Autodesk Inventor part; units mm, degrees
ref_plane "YZ Plane" through (0, 0, 0) normal (1, 0, 0) x (0, 1, 0)
ref_plane "XZ Plane" through (0, 0, 0) normal (0, 1, 0) x (-1, 0, 0)
ref_plane "XY Plane" through (0, 0, 0) normal (0, 0, 1) x (1, 0, 0)
sketch "Sketch1" plane through (0, 0, 0) normal (1, 0, 0) x (0, 1, 0)
  line L0 (0, 20) -> (6, 20) construction
  arc A0 (7.7498, 0) -> (6, 20) centre (-30.6677, 6.7154) ccw construction
  line L1 (0, 16) -> (0, 0) construction
  line L2 (6, 20) -> (2.4961, 20) construction
  line L3 (7.7498, 0) -> (4.5, 0) construction
  line L4 (4.5, 10) -> (0, 10)
  line L5 (4.5, 10) -> (4.5, 0)
  line L6 (0, 16) -> (0, 10)
  line L7 (7.7498, 0) -> (6, 20) construction
  line L8 (4.5, 0) -> (7.7498, 0)
  line L9 (7.7498, 0) -> (6, 20)
  line L10 (0, 16) -> (0.8, 16)
  line L11 (0.8, 16) -> (0.8, 20)
  line L12 (0.8, 20) -> (6, 20)
  dimension "d0" = 6
  dimension "d5" = 4.5
  dimension "d11" = 10
  dimension "d12" = 20
  dimension "d13" = 95
  dimension "d21" = 4
  dimension "d22" = 0.8
revolve "Revolution1" add sketch "Sketch1" angle 360 about axis through (0, 0, 16) along (0, 0, -1)
properties part number "brush fitting parta v4"
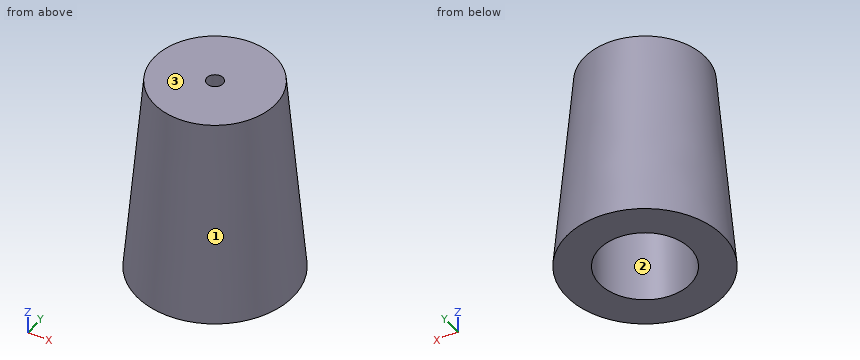
Design review of the part built by this model. Coordinates are the model's own, in mm. Face numbers are marked on the shaded views. Coordinates: 2 decimals unless noted, no trailing zeros. Order: outer loops, then holes, each group sorted by start corner. A loop starts at its lowest first (then second) coordinate and runs counter-clockwise, first axis right, second up.
1) Mouldability with a two-part tool opening along X and no side actions: class the marked faces 1, 2 and 3 as +X half, -X half, draft (parallel to the pull), parting line (faces both ways), or undercut.
2) Wall thickness on line 1 along Z through (x, y) = (1.5, 1.25); line 2 along X through (y, z) = (0, 18.6); line 3 along X through (y, z) = (0.5, 5.5): over which ranges is each line inside the solid? List them lowest first.
3) Take a section at A-A, the plane x = 0. Give the boundary of the cut face in (y, z), and give its area (3 significant figures).
4) Clearance check with flat-ended pins moving along their axes: pin 1 (1.5 mm diameter, centred on x = -6, z = 17, fed in from -Y); pin 2 (2 mm diameter, centred on x = -4.5, z = 6.5, fed in from +Y); pin 3 (2 mm diameter, centred on x = -3, z = 6.5, fed in from +Y). State where each tip first meets the part, or that it passes through.
5) Take a section at C-C, the plane z = 1.75. Give the boundary of the cut face in (x, y), and give its area (3 significant figures).
6) Take a section at D-D, the plane z = 18.5. Give the boundary of the cut face in (x, y), and give its area (3 significant figures).
Returned:
1. face 1: parting line
1. face 2: undercut
1. face 3: draft
2. line 1: z = 10 to 20
2. line 2: x = -6.12 to -0.8, 0.8 to 6.12
2. line 3: x = -7.25 to -4.47, 4.47 to 7.25
3. outline: (-7.75, 0) - (-4.5, 0) - (-4.5, 10) - (4.5, 10) - (4.5, 0) - (7.75, 0) - (6, 20) - (0.8, 20) - (0.8, 16) - (-0.8, 16) - (-0.8, 20) - (-6, 20) - close
3. area: 179 mm2
4. pin 1: stops at y = -3.42
4. pin 2: stops at y = 6.28
4. pin 3: stops at y = 6.91
5. outline: circle Ø15.19 at (0, 0); hole circle Ø9 at (0, 0)
5. area: 118 mm2
6. outline: circle Ø12.26 at (0, 0); hole circle Ø1.6 at (0, 0)
6. area: 116 mm2
